For this review, take the finished solid that the model builds, in its own axes (mm). Coordinates: 2 decimals unless noted, no trailing zeros. Write each loop counter-clockwise with the first axis right and the second up, starting at its lowest first coordinate (ties: lowest second). Pieces come first, ordered by that corner, then holes. Notation, with made-up numbers: (61, 58.25) -> (95, 58.25) arc R16 cw to (95, 71.25) -> close; hole circle Ø2 at (-10, 64.5). An arc over 180 degrees is marked (long way). Put each result on its own line as item: value. Start each with the question number.
Item 1: Consider section C-C on y = 2.5. Give the boundary of the cut face in (x, z), and give its area (3 significant figures).
Item 2: Consider section B-B on z = 0. Give the boundary of the cut face in (x, y).
Item 3: Consider section D-D on y = 4.5. Give the boundary of the cut face in (x, z), and give its area (3 significant figures).
Item 4: Insertion check: P1, Ø6, axis at x = 3.5, y = 2.5, coming from the -Z side; P2, Ø1, axis at y = 2.5, z = 5.5, coming from the +X side; P3, Ø2, axis at y = 3, z = -7.5, coming from the -X side. Each pin has a flat end and moves straight along its axis. Give the tip position at first contact, or say it passes through.
Item 5: To check wall thickness, follow L1, parallel to X at y = 1.25, z = 6.5; L2, parallel to Z at x = -1, y = -1.75; L3, parallel to X at y = 3, z = 6. State the ranges of each line that lie inside material, in increasing order.
Item 6: Consider section A-A on x = 0. Give the boundary of the cut face in (y, z).
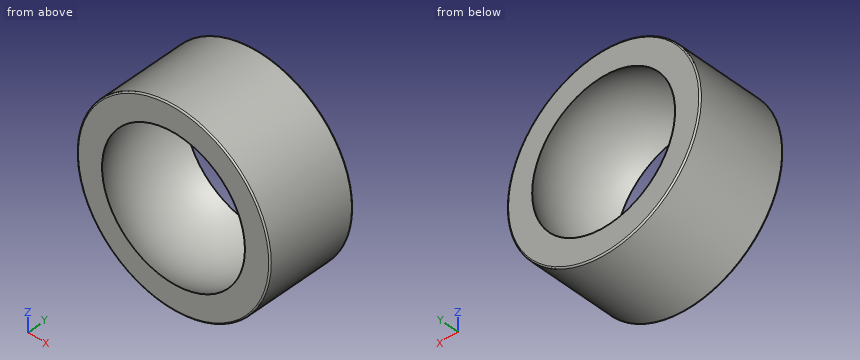
```python
from build123d import *

# Parameters (mm, degrees)
SZKIC1_R                    = 14.5
DODANIE_WYCI_GNI_CIE1_DEPTH = 6.75
ZAOKR_GLENIE1_R             = 0.2


with BuildPart() as part:
    # Szkic1 → Dodanie-wyciągnięcie1 (new body, symmetric)
    with BuildSketch(Plane(origin=(0, 0, 0), x_dir=(1, 0, 0), z_dir=(0, 1, 0))):
        Circle(SZKIC1_R)
    extrude(amount=DODANIE_WYCI_GNI_CIE1_DEPTH, both=True)

    # Szkic3 → Wycięcie-obrót1 (revolve, cut)
    with BuildSketch(Plane.XY):
        with BuildLine():
            Line((0, -12.68), (0, 12.68))
            ThreePointArc((0, 12.68), (12.68, 0), (0, -12.68))
        make_face()
    revolve(axis=Axis((0, -12.68, 0), (0, 1, 0)), mode=Mode.SUBTRACT)

    # Zaokrąglenie1
    zaokr_glenie1_edges = [part.edges().sort_by_distance(p)[0] for p in [
        (-14.5, -6.75, 0),
        (-14.5, 6.75, 0),
    ]]
    fillet(zaokr_glenie1_edges, radius=ZAOKR_GLENIE1_R)


solid = part.part
```
Return value:
1. outline: circle Ø29 at (0, 0); hole circle Ø24.86 at (0, 0)
1. area: 175 mm^2
2. outline: (-14.5, -6.55) arc R0.2 ccw to (-14.3, -6.75) -> (-10.73, -6.75) arc R12.68 cw to (-10.73, 6.75) -> (-14.3, 6.75) arc R0.2 ccw to (-14.5, 6.55) -> close; (10.73, -6.75) -> (14.3, -6.75) arc R0.2 ccw to (14.5, -6.55) -> (14.5, 6.55) arc R0.2 ccw to (14.3, 6.75) -> (10.73, 6.75) arc R12.68 cw to start
3. outline: circle Ø29 at (0, 0); hole circle Ø23.71 at (0, 0)
3. area: 219 mm^2
4. P1: z = -14.49
4. P2: x = 13.61
4. P3: x = -12.96
5. L1: -12.96 to -10.82, 10.82 to 12.96
5. L2: -14.47 to -12.52, 12.52 to 14.47
5. L3: -13.2 to -10.76, 10.76 to 13.2
6. outline: (-6.75, -14.3) arc R0.2 ccw to (-6.55, -14.5) -> (6.55, -14.5) arc R0.2 ccw to (6.75, -14.3) -> (6.75, -10.73) arc R12.68 cw to (-6.75, -10.73) -> close; (-6.75, 10.73) arc R12.68 cw to (6.75, 10.73) -> (6.75, 14.3) arc R0.2 ccw to (6.55, 14.5) -> (-6.55, 14.5) arc R0.2 ccw to (-6.75, 14.3) -> close
